```python
from build123d import *

# Parameters (mm, degrees)
F1_DEPTH = 70
F3_START = -25
F3_DEPTH = 50


with BuildPart() as f1:
    # F0 (on Front) → F1 (new body)
    with BuildSketch(Plane.XZ):
        with BuildLine():
            ThreePointArc((-21, -0.4), (-20, 0.1), (-19, -0.4))
            ThreePointArc((-19, -0.4), (-18, -0.9), (-17, -0.4))
            ThreePointArc((-17, -0.4), (-16, 0.1), (-15, -0.4))
            ThreePointArc((-15, -0.4), (-14, -0.9), (-13, -0.4))
            ThreePointArc((-13, -0.4), (-12, 0.1), (-11, -0.4))
            ThreePointArc((-11, -0.4), (-10, -0.9), (-9, -0.4))
            ThreePointArc((-9, -0.4), (-8, 0.1), (-7, -0.4))
            ThreePointArc((-7, -0.4), (-6, -0.9), (-5, -0.4))
            ThreePointArc((-5, -0.4), (-4, 0.1), (-3, -0.4))
            ThreePointArc((-3, -0.4), (-2, -0.9), (-1, -0.4))
            ThreePointArc((-1, -0.4), (0, 0.1), (1, -0.4))
            ThreePointArc((1, -0.4), (2, -0.9), (3, -0.4))
            ThreePointArc((3, -0.4), (4, 0.1), (5, -0.4))
            ThreePointArc((5, -0.4), (6, -0.9), (7, -0.4))
            ThreePointArc((7, -0.4), (8, 0.1), (9, -0.4))
            ThreePointArc((9, -0.4), (10, -0.9), (11, -0.4))
            ThreePointArc((11, -0.4), (12, 0.1), (13, -0.4))
            ThreePointArc((13, -0.4), (14, -0.9), (15, -0.4))
            ThreePointArc((15, -0.4), (16, 0.1), (17, -0.4))
            ThreePointArc((17, -0.4), (18, -0.9), (19, -0.4))
            ThreePointArc((19, -0.4), (20, 0.1), (21, -0.4))
            ThreePointArc((21, -0.4), (22, -0.9), (23, -0.4))
            ThreePointArc((23, -0.4), (24, 0.1), (25, -0.4))
            Line((25, -0.4), (25, 0.4))
            ThreePointArc((25, 0.4), (24, 0.9), (23, 0.4))
            ThreePointArc((23, 0.4), (22, -0.1), (21, 0.4))
            ThreePointArc((21, 0.4), (20, 0.9), (19, 0.4))
            ThreePointArc((19, 0.4), (18, -0.1), (17, 0.4))
            ThreePointArc((17, 0.4), (16, 0.9), (15, 0.4))
            ThreePointArc((15, 0.4), (14, -0.1), (13, 0.4))
            ThreePointArc((13, 0.4), (12, 0.9), (11, 0.4))
            ThreePointArc((11, 0.4), (10, -0.1), (9, 0.4))
            ThreePointArc((9, 0.4), (8, 0.9), (7, 0.4))
            ThreePointArc((7, 0.4), (6, -0.1), (5, 0.4))
            ThreePointArc((5, 0.4), (4, 0.9), (3, 0.4))
            ThreePointArc((3, 0.4), (2, -0.1), (1, 0.4))
            ThreePointArc((1, 0.4), (0, 0.9), (-1, 0.4))
            ThreePointArc((-1, 0.4), (-2, -0.1), (-3, 0.4))
            ThreePointArc((-3, 0.4), (-4, 0.9), (-5, 0.4))
            ThreePointArc((-5, 0.4), (-6, -0.1), (-7, 0.4))
            ThreePointArc((-7, 0.4), (-8, 0.9), (-9, 0.4))
            ThreePointArc((-9, 0.4), (-10, -0.1), (-11, 0.4))
            ThreePointArc((-11, 0.4), (-12, 0.9), (-13, 0.4))
            ThreePointArc((-13, 0.4), (-14, -0.1), (-15, 0.4))
            ThreePointArc((-15, 0.4), (-16, 0.9), (-17, 0.4))
            ThreePointArc((-17, 0.4), (-18, -0.1), (-19, 0.4))
            ThreePointArc((-19, 0.4), (-20, 0.9), (-21, 0.4))
            ThreePointArc((-21, 0.4), (-22, -0.1), (-23, 0.4))
            ThreePointArc((-23, 0.4), (-24, 0.9), (-25, 0.4))
            Line((-25, 0.4), (-25, -0.4))
            ThreePointArc((-25, -0.4), (-24, 0.1), (-23, -0.4))
            ThreePointArc((-23, -0.4), (-22, -0.9), (-21, -0.4))
        make_face()
    extrude(amount=F1_DEPTH)

    # F2 (on Top) → F3 (intersect)
    with BuildSketch(Plane.XY.offset(F3_START)):
        with BuildLine():
            ThreePointArc((-12, -254.0961094374), (152.1248608016, -289.1042774324), (246, -150))
            ThreePointArc((246, -150), (152.1248608016, -10.8957225676), (-12, -45.9038905626))
            Line((-12, -45.9038905626), (-12, -150))
            Line((-12, -150), (-12, -254.0961094374))
        make_face()
    extrude(amount=F3_DEPTH, mode=Mode.INTERSECT)


solid = f1.part
```
Model file for the job. Use its own axes, mm. Coordinates: 2 decimals unless noted, no trailing zeros. Order: outer loops, then holes, each group sorted by start corner. A loop starts at its lowest first (then second) coordinate and runs counter-clockwise, first axis right, second up. Notation, with made-up numbers: (11.5, -30.75) -> (30.5, -30.75) arc R7 ccw to (30.5, -17.75) -> close; hole circle Ø9 at (-0.75, -21). An arc over 180 degrees is marked (long way). Return JSON: item names as keys, results as strings.
Item 1: Slice it at A-A (y = -31.5). Write the cut outline in (x, z), then the cut area to 3 significant figures.
Model answer:
{"outline": "(4.03, 0.1) arc R1.25 cw to (5, -0.4) arc R1.25 ccw to (7, -0.4) arc R1.25 cw to (9, -0.4) arc R1.25 ccw to (11, -0.4) arc R1.25 cw to (13, -0.4) arc R1.25 ccw to (15, -0.4) arc R1.25 cw to (17, -0.4) arc R1.25 ccw to (19, -0.4) arc R1.25 cw to (21, -0.4) arc R1.25 ccw to (23, -0.4) arc R1.25 cw to (25, -0.4) -> (25, 0.4) arc R1.25 ccw to (23, 0.4) arc R1.25 cw to (21, 0.4) arc R1.25 ccw to (19, 0.4) arc R1.25 cw to (17, 0.4) arc R1.25 ccw to (15, 0.4) arc R1.25 cw to (13, 0.4) arc R1.25 ccw to (11, 0.4) arc R1.25 cw to (9, 0.4) arc R1.25 ccw to (7, 0.4) arc R1.25 cw to (5, 0.4) arc R1.25 ccw to (4.03, 0.9) -> close", "area": "16.8 mm²"}
Item 2: Pin check, flat tip, straight feed: P1, Ø1.5, axis at x = 9, y = -46.5, coming from the -Z side. Stop position of the tip, or through.
Model answer:
{"P1": "stops at z = -0.87"}
Item 3: Wall check: line 1 along X through (y, z) = (-31.5, 0.7); line 2 along Z through (x, y) = (-1, -64.5); line 3 along Y through (x, z) = (23, -0.05). Give the ranges that are in metal, low to high. Write a range as from..to.
Model answer:
{"line 1": "x = 4.03..4.68, 7.32..8.68, 11.32..12.68, 15.32..16.68, 19.32..20.68, 23.32..24.68", "line 2": "z = -0.4..0.4", "line 3": "y = -70..-18.96"}
Item 4: Mould opens along X. For faces 1 (the face through (5.67, -30.25, -0.42)), 2 (the face through (6.2, -70, -0.4)) say: pulls with the +X half, pulls with the -X half, needs draft (parallel to the pull), parting line crosses it, or undercut.
Model answer:
{"face 1": "pulls with the -X half", "face 2": "needs draft"}
Item 5: Slice it at B-B (x = -2). Write the cut outline in (y, z), then the cut area to 3 significant figures.
Model answer:
{"outline": "(-70, -0.9) -> (-36.44, -0.9) -> (-36.44, -0.1) -> (-70, -0.1) -> close", "area": "26.8 mm²"}
